```python
from build123d import *

# Parameters (mm, degrees)
SKETCH_1_W              = 75
SKETCH_1_H              = 65
EXTRUDE_1_DEPTH         = 2
HOLE_WIZARD_4_4_4_4_1_D = 4.4
HOLE_WIZARD_2_5_2_5_1_D = 2.5
FILLET_1_R              = 4
SKETCH_6_W              = 45
SKETCH_6_H              = 26
CUT_EXTRUDE_1_DEPTH     = 50.663870167
FILLET_2_R              = 4


with BuildPart() as part:
    # 草图1 → 凸台-拉伸1 (new body)
    with BuildSketch(Plane(origin=(0, 0, 0), x_dir=(1, 0, 0), z_dir=(0, 1, 0))):
        Rectangle(SKETCH_1_W, SKETCH_1_H)
    extrude(amount=EXTRUDE_1_DEPTH)

    # Ø4.4 (4.4) 直径孔1 (through all)
    with Locations(Plane(origin=(-32.5, 2, -22.5), x_dir=(0, 0, 1), z_dir=(0, 1, 0))):
        with Locations((0, 0), (0, 65)):
            Hole(HOLE_WIZARD_4_4_4_4_1_D / 2)

    # Ø2.5 (2.5) 直径孔1 (through all)
    with Locations(Plane(origin=(-18, 2, -7.5), x_dir=(0, 0, 1), z_dir=(0, 1, 0))):
        with Locations((0, 0), (36, 0)):
            hole_wizard_2_5_2_5_1 = Hole(HOLE_WIZARD_2_5_2_5_1_D / 2)

    # 镜向1: Ø2.5 (2.5) 直径孔1 across plane
    add(hole_wizard_2_5_2_5_1.mirror(Plane(origin=(0, 0, 0), x_dir=(0, 0, 1), z_dir=(1, 0, 0))), mode=Mode.SUBTRACT)

    # 圆角1
    fillet_1_edges = [part.edges().sort_by_distance(p)[0] for p in [
        (37.5, 1, 32.5),
        (-37.5, 1, 32.5),
        (-37.5, 1, -32.5),
        (37.5, 1, -32.5),
    ]]
    fillet(fillet_1_edges, radius=FILLET_1_R)

    # 草图6 → 切除-拉伸1 (cut, through all)
    with BuildSketch(Plane(origin=(0, 2, 0), x_dir=(1, 0, 0), z_dir=(0, 1, 0))):
        with Locations((0, -10.5)):
            Rectangle(SKETCH_6_W, SKETCH_6_H)
    extrude(amount=-CUT_EXTRUDE_1_DEPTH, mode=Mode.SUBTRACT)

    # 圆角2
    fillet_2_edges = [part.edges().sort_by_distance(p)[0] for p in [
        (-22.5, 1, 23.5),
        (-22.5, 1, -2.5),
        (22.5, 1, -2.5),
        (22.5, 1, 23.5),
    ]]
    fillet(fillet_2_edges, radius=FILLET_2_R)


solid = part.part
```
Geometry check sheet. Reference: the model listing, model coordinates, mm. A direction names the side the tool comes from. Coordinates: 2 decimals unless noted, no trailing zeros. Write each loop counter-clockwise with the first axis right and the second up, starting at its lowest first coordinate (ties: lowest second). Pieces come first, ordered by that corner, then holes. Notation, with made-up numbers: M -1,49.5 L 21,49.5 A27 cw 21,78.5 Z; hole C 40,85.25 d9. An arc over 180 degrees is marked long. One line per item, written item: value. Start each with the question number.
(1) Scan lines: line 1 along X through (y, z) = (1.6, -22.5); line 2 along X through (y, z) = (1.6, -7.5); line 3 along Z through (x, y) = (-10, 0.85). Record each from-to range of solid material in increasing order. Write a range as [from, to].
(2) Release check for a two-part mould opening along Z. For faces 1 (the face through (0, 1, -32.5)), 2 (the face through (-1, 0, -8)), 3 (the face through (30.352, 0.986, -22.023)), 4 (the face through (-22.5, 1, 11)) record: released by +Z, released by -Z, zero draft, split by the parting line, or undercut.
(3) Sectioned sample at B-B, the plane z = 16.5. Enter the section's corners in (x, y), and give its area (3 significant figures).
(4) Sectioned sample at C-C, the plane y = 1.5. Enter the section's corners in (x, z).
(5) Sectioned sample at A-A, the plane x = 32.5. Enter the section's corners in (y, z).
(6) Tool access check on faces 5 (the face through (0, 1, 32.5)), 6 (the face through (21.297, 0.986, 22.359)). Record the directions out of +Z, -Z, +X, -X, +Y, -Y that give a thin tool (end or side, any length) a straight path to the whole face; none if there is none.
(7) Depth check by flat-ended pin: pin 1 (5 mm diameter, centred on x = -32.5, z = -22.5, fed in from +Y). Enter the tip coordinate at first touch or a pass-through.
(8) Sectioned sample at D-D, the plane z = -7.5. Enter the section's corners in (x, y), and give its area (3 significant figures).
Filled sheet:
1. line 1: [-37.5, -34.7], [-30.3, 30.3], [34.7, 37.5]
1. line 2: [-37.5, -19.25], [-16.75, 16.75], [19.25, 37.5]
1. line 3: [-32.5, -2.5], [23.5, 32.5]
2. face 1: released by -Z
2. face 2: zero draft
2. face 3: undercut
2. face 4: undercut
3. outline: M -37.5,0 L -22.5,0 L -22.5,2 L -37.5,2 Z; M 22.5,0 L 37.5,0 L 37.5,2 L 22.5,2 Z
3. area: 60.0 mm²
4. outline: M -37.5,-28.5 A4 ccw -33.5,-32.5 L 33.5,-32.5 A4 ccw 37.5,-28.5 L 37.5,28.5 A4 ccw 33.5,32.5 L -33.5,32.5 A4 ccw -37.5,28.5 Z; hole C -32.5,-22.5 d4.4; hole M -22.5,1.5 A4 ccw -18.5,-2.5 L 18.5,-2.5 A4 ccw 22.5,1.5 L 22.5,19.5 A4 ccw 18.5,23.5 L -18.5,23.5 A4 ccw -22.5,19.5 Z; hole C -18,-7.5 d2.5; hole C -18,28.5 d2.5; hole C 18,-7.5 d2.5; hole C 18,28.5 d2.5; hole C 32.5,-22.5 d4.4
5. outline: M 0,-32.5 L 2,-32.5 L 2,-24.7 L 0,-24.7 Z; M 0,-20.3 L 2,-20.3 L 2,32.5 L 0,32.5 Z
6. face 5: +Z, +X, -X, +Y, -Y
6. face 6: +Y, -Y
7. pin 1: y = 2
8. outline: M -37.5,0 L -19.25,0 L -19.25,2 L -37.5,2 Z; M -16.75,0 L 16.75,0 L 16.75,2 L -16.75,2 Z; M 19.25,0 L 37.5,0 L 37.5,2 L 19.25,2 Z
8. area: 140 mm²
